Model file for the job. Use its own axes, mm. Face numbers are marked on the shaded views. A direction names the side the tool comes from. Round coordinates to 2 decimals unless told otherwise and drop trailing zeros. Write each loop counter-clockwise with the first axis right and the second up, starting at its lowest first coordinate (ties: lowest second). Pieces come first, ordered by that corner, then holes. Notation, with made-up numbers: (79, 33.25) - (95, 33.25) arc R19 ccw to (95, 45.25) - close; hole circle Ø9 at (72.5, 70.25). An arc over 180 degrees is marked (long way). Answer as a JSON object with one key per item and string values. Group by question number.
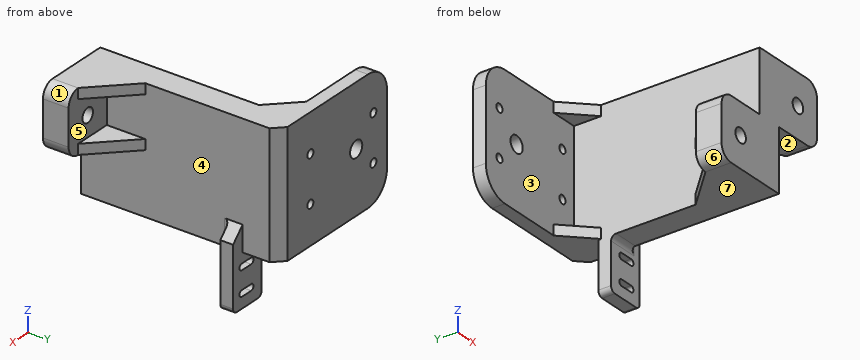
from build123d import *

# Parameters (mm, degrees)
SKETCH1_W                 = 56.15
SKETCH1_H                 = 48
BOSS_EXTRUDE1_DEPTH       = 5
SKETCH2_W                 = 10
SKETCH2_H                 = 48
BOSS_EXTRUDE2_DEPTH       = 72.5
SKETCH3_W                 = 24
SKETCH3_H                 = 10
BOSS_EXTRUDE3_DEPTH       = 20
SKETCH20_W                = 24
SKETCH20_H                = 10
BOSS_EXTRUDE5_DEPTH       = 20
FILLET1_R                 = 10
F_1_0MM_DOWEL_HOLE1_D     = 5.5
F_1_0MM_DOWEL_HOLE1_DEPTH = 10
FILLET2_R                 = 5
RIB1_REACH                = 103.39
SKETCH19_WALL_W           = 225.992615606
SKETCH19_WALL_H           = 4
M3_CLEARANCE_HOLE1_D      = 3.2
M3_CLEARANCE_HOLE1_DEPTH  = 5
M6_CLEARANCE_HOLE1_D      = 6.4
CHAMFER2_SIZE             = 4
SKETCH14_W                = 15
SKETCH14_H                = 5
BOSS_EXTRUDE4_DEPTH       = 20
CHAMFER3_SIZE             = 10
FILLET3_R                 = 2
M2_START                  = -14.5
M2_CLEARANCE_SLOT2_DEPTH  = 5
RIB5_REACH                = 103.39
SKETCH21_WALL_W           = 225.992615606
SKETCH21_WALL_H           = 4
BOSS_EXTRUDE6_DEPTH       = 4


# Read off the part's stored shape, not the designer's step: M2 Clearance Slot2
with BuildPart() as part:
    # Sketch1 → Boss-Extrude1 (new body)
    with BuildSketch(Plane(origin=(0, 0, 0), x_dir=(1, 0, 0), z_dir=(0, 1, 0))):
        with Locations((4.075, 0)):
            Rectangle(SKETCH1_W, SKETCH1_H)
    extrude(amount=BOSS_EXTRUDE1_DEPTH)

    # Sketch2 → Boss-Extrude2 (add)
    with BuildSketch(Plane.XZ):
        with Locations((27.15, 0)):
            Rectangle(SKETCH2_W, SKETCH2_H)
    extrude(amount=BOSS_EXTRUDE2_DEPTH)

    # Sketch3 → Boss-Extrude3 (add)
    with BuildSketch(Plane(origin=(32.15, 0, 0), x_dir=(0, 0, -1), z_dir=(1, 0, 0))):
        with Locations((-12, -67.5)):
            Rectangle(SKETCH3_W, SKETCH3_H)
    extrude(amount=BOSS_EXTRUDE3_DEPTH)

    # Sketch20 → Boss-Extrude5 (add)
    with BuildSketch(Plane.ZY.offset(-22.15)):
        with Locations((-12, -67.5)):
            Rectangle(SKETCH20_W, SKETCH20_H)
    extrude(amount=BOSS_EXTRUDE5_DEPTH)

    # Fillet1
    fillet1_edges = [part.edges().sort_by_distance(p)[0] for p in [
        (-24, 2.5, -24),
        (-24, 2.5, 24),
    ]]
    fillet(fillet1_edges, radius=FILLET1_R)

    # Ø1.0mm Dowel Hole1
    with Locations(Plane(origin=(0, -62.5, 0), x_dir=(1, 0, 0), z_dir=(0, 1, 0))):
        with Locations((42.15, -12), (12.15, 12)):
            Hole(F_1_0MM_DOWEL_HOLE1_D / 2, depth=F_1_0MM_DOWEL_HOLE1_DEPTH)

    # Fillet2
    fillet2_edges = [part.edges().sort_by_distance(p)[0] for p in [
        (52.15, -67.5, 24),
        (52.15, -67.5, 0),
        (2.15, -67.5, -24),
        (2.15, -67.5, 0),
    ]]
    fillet(fillet2_edges, radius=FILLET2_R)

    # Sketch19 wall → Rib1 (add, up to next)
    with BuildSketch(Plane(origin=(39.65, -55, 24), x_dir=(0.707106781187, -0.707106781187, 0), z_dir=(0.707106781187, 0.707106781187, 0)), mode=Mode.PRIVATE) as rib1_sk1:
        with Locations((0, 2)):
            Rectangle(SKETCH19_WALL_W, SKETCH19_WALL_H)
    rib1_tool1 = extrude(rib1_sk1.sketch, amount=-RIB1_REACH, mode=Mode.PRIVATE) - part.part
    rib1 = rib1_tool1.solids().sort_by_distance((39.65, -55, 24))[0]
    add(rib1)

    # M3 Clearance Hole1
    with Locations(Plane(origin=(0, 5, 0), x_dir=(1, 0, 0), z_dir=(0, 1, 0))):
        with Locations((-16.85, -9), (-16.85, 9), (16.15, 9), (16.15, -9)):
            Hole(M3_CLEARANCE_HOLE1_D / 2, depth=M3_CLEARANCE_HOLE1_DEPTH)

    # M6 Clearance Hole1 (through all)
    with Locations(Plane(origin=(0, 5, 0), x_dir=(1, 0, 0), z_dir=(0, 1, 0))):
        with Locations((-7.85, 0)):
            Hole(M6_CLEARANCE_HOLE1_D / 2)

    # Chamfer2
    chamfer2_edges = [part.edges().sort_by_distance(p)[0] for p in [
        (32.15, 5, 0),
    ]]
    chamfer(chamfer2_edges, length=CHAMFER2_SIZE)

    # Sketch14 → Boss-Extrude4 (add)
    with BuildSketch(Plane(origin=(0, 0, -24), x_dir=(-1, 0, 0), z_dir=(0, 0, -1))):
        with Locations((-29.65, -12)):
            Rectangle(SKETCH14_W, SKETCH14_H)
    extrude(amount=BOSS_EXTRUDE4_DEPTH)

    # Chamfer3
    # the kernel refuses this chamfer: 10 mm, written as the material it adds along each edge
    with BuildSketch(Plane(origin=(32.15, -9.5, -24), x_dir=(-0.027495876610586317, 0, 0.9996219169112968), z_dir=(0, -1, 0))) as chamfer3_piece_1_section:
        Polygon((CHAMFER3_SIZE * 0.999621916911, -CHAMFER3_SIZE * 0.0274958766106), (-CHAMFER3_SIZE * 0.0274958766106, -CHAMFER3_SIZE * 0.999621916911), (0, 0), align=None)
    chamfer3_piece_1 = extrude(amount=5, mode=Mode.PRIVATE)
    chamfer3_piece_1 = split(chamfer3_piece_1, bisect_by=Plane(origin=(37.15, -12, -20.111111111), z_dir=(-1, 0, 0)), keep=Keep.TOP, mode=Mode.PRIVATE)
    add(chamfer3_piece_1)

    # Fillet3
    fillet3_edges = [part.edges().sort_by_distance(p)[0] for p in [
        (27.15, -14.5, -24),
        (22.15, -12, -44),
        (37.15, -12, -44),
        (32.15, -14.5, -19),
    ]]
    fillet(fillet3_edges, radius=FILLET3_R)

    # M2 Clearance Slot2 outline → M2 Clearance Slot2 (cut)
    with BuildSketch(Plane(origin=(0, 0, 0), x_dir=(1, 0, 0), z_dir=(0, 1, 0)).offset(M2_START)):
        with BuildLine():
            Line((32.65, 39.7), (27.65, 39.7))
            ThreePointArc((27.65, 39.7), (26.45, 38.5), (27.65, 37.3))
            Line((27.65, 37.3), (32.65, 37.3))
            ThreePointArc((32.65, 37.3), (33.85, 38.5), (32.65, 39.7))
        make_face()
        with BuildLine():
            ThreePointArc((32.65, 27.8), (33.85, 29), (32.65, 30.2))
            Line((32.65, 30.2), (27.65, 30.2))
            ThreePointArc((27.65, 30.2), (26.45, 29), (27.65, 27.8))
            Line((27.65, 27.8), (32.65, 27.8))
        make_face()
    extrude(amount=M2_CLEARANCE_SLOT2_DEPTH, mode=Mode.SUBTRACT)

    # Mirror1: Rib1 across plane
    add(rib1.mirror(Plane(origin=(52.15, -62.5, 12), x_dir=(1, 0, 0), z_dir=(0, 0, -1))))

    # Sketch21 wall → Rib5 (add, up to next)
    with BuildSketch(Plane(origin=(14.65, -55, -24), x_dir=(-0.707106781187, -0.707106781187, 0), z_dir=(-0.707106781187, 0.707106781187, 0)), mode=Mode.PRIVATE) as rib5_sk1:
        with Locations((0, 2)):
            Rectangle(SKETCH21_WALL_W, SKETCH21_WALL_H)
    rib5_tool1 = extrude(rib5_sk1.sketch, amount=-RIB5_REACH, mode=Mode.PRIVATE) - part.part
    rib5 = rib5_tool1.solids().sort_by_distance((14.65, -55, -24))[0]
    add(rib5)

    # Mirror2: Rib5 across plane
    add(rib5.mirror(Plane(origin=(2.15, -62.5, -12), x_dir=(1, 0, 0), z_dir=(0, 0, 1))))

    # Sketch24 → Boss-Extrude6 (add)
    with BuildSketch(Plane.XY.offset(24)):
        Polygon((11.543398282, 0), (22.15, -10.606601718), (22.15, 0), align=None)
    boss_extrude6 = extrude(amount=-BOSS_EXTRUDE6_DEPTH)

    # Mirror3: Boss-Extrude6 across plane
    add(boss_extrude6.mirror(Plane.XY))


solid = part.part
(1) Slice it at B-B (z = -38.5). Write the cut outline in (x, y).
(2) Drill centre lines: line 1 (X direction, y = 1, z = 9); line 2 (Z direction, x = 42.15, y = -66.5); line 3 (Z direction, x = 16.15, y = 1.65). Where is each one in solid material? Low to high. Write a range as from..to.
(3) Pull direction Z, two halves, no side cores. Call the marked faces 1, 2 and 3: pulls with the +Z half, pulls with the -Z half, needs draft (parallel to the pull), parting line crosses it, or undercut.
(4) Slice it at C-C (x = -16.85). Write the cut outline in (y, z).
(5) Slice it at A-A (x = 42.15). Write the cut outline in (y, z).
(6) Slice it at D-D (y = -58). Write the cut outline in (x, z).
(7) 3-axis set-ups, long thin cutter, end or side, ignore diameter. For the marked faces 4, 5, 6 and 7: which of +Z, -Z, +X, -X, +Y, -Y reach the whole face in a straight line?
(8) Flat gauge pins, fed straight in: pin 1 (12 mm diameter, centred on y = -17, z = 15.5, fed in from -X); pin 2 (12 mm diameter, centred on y = -26, z = 14, fed in from -X); pin 3 (7.5 mm diameter, centred on x = 17, y = -53, fed in from +Z). Where does each tip first touch, or does it go through?
Answer:
{
 "1": {"outline": "(22.15, -14.5) - (26.45, -14.5) - (26.45, -9.5) - (22.15, -9.5) - close; (33.85, -14.5) - (37.15, -14.5) - (37.15, -9.5) - (33.85, -9.5) - close"},
 "2": {"line 1": "-24..-18.45, -15.25..14.55, 17.75..32.15", "line 2": "0..9.25, 14.75..24", "line 3": "-24..-10.6, -7.4..7.4, 10.6..24"},
 "3": {"face 1": "pulls with the +Z half", "face 2": "pulls with the -Z half", "face 3": "undercut"},
 "4": {"outline": "(0, -23.59) - (5, -23.59) - (5, -10.6) - (0, -10.6) - close; (0, -7.4) - (5, -7.4) - (5, 7.4) - (0, 7.4) - close; (0, 10.6) - (5, 10.6) - (5, 23.59) - (0, 23.59) - close"},
 "5": {"outline": "(-72.5, 0) - (-57.5, 0) - (-57.5, 4) - (-62.5, 4) - (-62.5, 9.25) - (-72.5, 9.25) - close; (-72.5, 14.75) - (-62.5, 14.75) - (-62.5, 20) - (-57.5, 20) - (-57.5, 24) - (-72.5, 24) - close"},
 "6": {"outline": "(11.65, -24) - (32.15, -24) - (32.15, 0) - (42.65, 0) - (42.65, 4) - (32.15, 4) - (32.15, 20) - (42.65, 20) - (42.65, 24) - (22.15, 24) - (22.15, 0) - (11.65, 0) - (11.65, -4) - (22.15, -4) - (22.15, -20) - (11.65, -20) - close"},
 "7": {"face 4": "+X", "face 5": "+X, +Y", "face 6": "-Z, -X, -Y", "face 7": "-Z, +X, -X, -Y"},
 "8": {"pin 1": "x = 22.15", "pin 2": "x = 22.15", "pin 3": "z = 0"}
}
